from build123d import *

# Parameters (mm, degrees)
SKETCH1_R           = 7.9375
OUTER_CIRCLE_DEPTH  = 6.35
TOOTH_CUT_DEPTH     = 13.896910967
TEETH_PATTERN_COUNT = 18
SKETCH3_R           = 1.56718
CUT_EXTRUDE1_DEPTH  = 13.857185215


with BuildPart() as part:
    # Sketch1 → Outer Circle (new body)
    with BuildSketch(Plane.XY):
        Circle(SKETCH1_R)
    extrude(amount=OUTER_CIRCLE_DEPTH)

    # Sketch2 → Tooth Cut (cut, through all)
    with BuildSketch(Plane.XY.offset(6.35)):
        with BuildLine():
            ThreePointArc((-0.452232993, 6.333876011), (0, 6.35), (0.452232993, 6.333876011))
            ThreePointArc((0.452232993, 6.333876011), (0.624488533, 7.142351531), (1.011484471, 7.872788922))
            ThreePointArc((1.011484471, 7.872788922), (0, 7.9375), (-1.011484471, 7.872788922))
            ThreePointArc((-1.011484471, 7.872788922), (-0.624488533, 7.142351531), (-0.452232993, 6.333876011))
        make_face()
    tooth_cut = extrude(amount=-TOOTH_CUT_DEPTH, mode=Mode.SUBTRACT)

    # Teeth Pattern: Tooth Cut ×18 about axis
    teeth_pattern_axis = Axis((0, 0, 0), (0, 0, 1))
    for i in range(1, TEETH_PATTERN_COUNT):
        add(tooth_cut.rotate(teeth_pattern_axis, i * 360 / TEETH_PATTERN_COUNT), mode=Mode.SUBTRACT)

    # Sketch3 → Cut-Extrude1 (cut, through all)
    with BuildSketch(Plane(origin=(0, 0, 0), x_dir=(-1, 0, 0), z_dir=(0, 0, -1))):
        Circle(SKETCH3_R)
    extrude(amount=-CUT_EXTRUDE1_DEPTH, mode=Mode.SUBTRACT)


solid = part.part
CAD build for the part. Positions are in the model's coordinates, mm. A direction names the side the tool comes from. Coordinates: 2 decimals unless noted, no trailing zeros. Write each loop counter-clockwise with the first axis right and the second up, starting at its lowest first coordinate (ties: lowest second). Pieces come first, ordered by that corner, then holes. Notation, with made-up numbers: M 79,81 L 95,81 A35 cw 95,118 Z; hole C 3.5,-30.75 d4. An arc over 180 degrees is marked long. Return JSON: item names as keys, results as strings.
Item 1: Slice it at B-B, the plane x = 0. Write the cut outline in (y, z), and give its area (3 significant figures).
Findings below:
{"outline": "M -6.35,0 L -1.57,0 L -1.57,6.35 L -6.35,6.35 Z; M 1.57,0 L 6.35,0 L 6.35,6.35 L 1.57,6.35 Z", "area": "60.7 mm2"}
Item 2: Drop flat-ended pins along their axis: pin 1 Ø1 at (y, z) = (2, 2.5) entering from +X; pin 2 Ø3 at (x, z) = (3.5, 5.5) entering from -Y; pin 3 Ø3 at (y, z) = (5, 5) entering from -X. Give the stop position or say it passes through.
Findings below:
{"pin 1": "stops at x = 7.58", "pin 2": "stops at y = -7.05", "pin 3": "stops at x = -6.31"}
Item 3: Probe line 1 (X direction, y = -6.5, z = 4.5); line 2 (Y direction, x = 0, z = 1.5); line 3 (Y direction, x = 0.25, z = 6). List the from-to ranges inside material, lowest first. Write a range as from..to.
Findings below:
{"line 1": "x = -4.27..-3.03, -1.83..-0.47, 0.47..1.83, 3.03..4.27", "line 2": "y = -6.35..-1.57, 1.57..6.35", "line 3": "y = -6.35..-1.55, 1.55..6.35"}
Item 4: Which spindle directions (+Z, -Z, +X, -X, +Y, -Y) get a long thin tool onto all of the face, cutting with end or side? Do faces 1 (the cylindrical face through (5.866, -4.103, 3.219)), 2 (the cylindrical face through (-7.154, 0.623, 3.219)), 3 (the cylindrical face through (-3.04, 6.51, 3.22)), 4 (the cylindrical face through (0.01, -6.35, 3.22)). Say none if no direction does.
Findings below:
{"face 1": "+Z, -Z, +X", "face 2": "+Z, -Z", "face 3": "+Z, -Z, +Y", "face 4": "+Z, -Z, -Y"}
Item 5: Slice it at C-C, the plane y = 2. Write the cut outline in (x, z).
Findings below:
{"outline": "M -7.15,0 L 7.15,0 L 7.15,6.35 L -7.15,6.35 Z"}
Item 6: Two-plate mould, pull along X, no slides. Class faces 5 (the cylindrical face through (-3.022, -6.489, 3.219)), 6 (the cylindrical face through (-5.866, 4.103, 3.219)), 7 (the flat face through (0, -2, 0)): +X half, -X half, draft (parallel to the pull), parting line (faces both ways), or undercut.
Findings below:
{"face 5": "undercut", "face 6": "-X half", "face 7": "draft"}
Item 7: Slice it at A-A, the plane y = 0. Write the cut outline in (x, z).
Findings below:
{"outline": "M -7.94,0 L -1.57,0 L -1.57,6.35 L -7.94,6.35 Z; M 1.57,0 L 7.94,0 L 7.94,6.35 L 1.57,6.35 Z"}
